```python
from build123d import *
from OCP.BRepFilletAPI import BRepFilletAPI_MakeChamfer

# Parameters (mm, degrees)
BOSS_EXTRUDE1_DEPTH = 16.9
BOSS_EXTRUDE2_DEPTH = 13.5
BOSS_EXTRUDE3_DEPTH = 3.4
BOSS_EXTRUDE4_DEPTH = 13.5
CUT_EXTRUDE1_DEPTH  = 46.31468443
CHAMFER1_SIZE       = 2
CHAMFER1_SIZE2      = 1.154700538
CUT_EXTRUDE2_DEPTH  = 47.441152279
FILLET1_R           = 0.5
SKETCH10_W          = 25
SKETCH10_H          = 28.6
CUT_EXTRUDE3_DEPTH  = 47.441152315


with BuildPart() as part:
    # Sketch1 → Boss-Extrude1 (new body)
    with BuildSketch(Plane.XY):
        Polygon((-20, -13.3), (20, -13.3), (20, 13.3), (-20, 13.3), (-20, 14.3), (21, 14.3), (21, -14.3), (-20, -14.3), align=None)
    extrude(amount=BOSS_EXTRUDE1_DEPTH)

    # Sketch4 → Boss-Extrude2 (add)
    with BuildSketch(Plane(origin=(0, 0, 0), x_dir=(-1, 0, 0), z_dir=(0, 0, -1))):
        with BuildLine():
            Line((-21, 4.825), (-36, 4.825))
            ThreePointArc((-36, 4.825), (-38.610615349, 4.05774722), (-40.390970849, 2))
            Line((-40.390970849, 2), (-30.875, 2))
            Line((-30.875, 2), (-30.875, -2))
            Line((-30.875, -2), (-40.390970849, -2))
            ThreePointArc((-40.390970849, -2), (-38.610615349, -4.05774722), (-36, -4.825))
            Line((-36, -4.825), (-21, -4.825))
            Line((-21, -4.825), (-21, 4.825))
        make_face()
    extrude(amount=-BOSS_EXTRUDE2_DEPTH)

    # Sketch5 → Boss-Extrude3 (add)
    with BuildSketch(Plane.XY.offset(13.5)):
        with BuildLine():
            Line((21, 4.825), (21, -4.825))
            Line((21, -4.825), (36, -4.825))
            ThreePointArc((36, -4.825), (38.610615349, -4.05774722), (40.390970849, -2))
            ThreePointArc((40.390970849, -2), (40.825, 0), (40.390970849, 2))
            ThreePointArc((40.390970849, 2), (38.610615349, 4.05774722), (36, 4.825))
            Line((36, 4.825), (21, 4.825))
        make_face()
    extrude(amount=BOSS_EXTRUDE3_DEPTH)

    # Sketch8 → Boss-Extrude4 (add)
    with BuildSketch(Plane(origin=(0, 0, 0), x_dir=(-1, 0, 0), z_dir=(0, 0, -1))):
        with BuildLine():
            Line((-37.5, 2), (-40.390970849, 2))
            ThreePointArc((-40.390970849, 2), (-40.825, 0), (-40.390970849, -2))
            Line((-40.390970849, -2), (-37.5, -2))
            ThreePointArc((-37.5, -2), (-38.5, 0), (-37.5, 2))
        make_face()
        with BuildLine():
            Line((-34.5, 2), (-30.875, 2))
            Line((-30.875, 2), (-30.875, -2))
            Line((-30.875, -2), (-34.5, -2))
            ThreePointArc((-34.5, -2), (-33.5, 0), (-34.5, 2))
        make_face()
    extrude(amount=-BOSS_EXTRUDE4_DEPTH)

    # Sketch9 → Cut-Extrude1 (cut, through all)
    with BuildSketch(Plane(origin=(0, 0, 13.5), x_dir=(-1, 0, 0), z_dir=(0, 0, -1))):
        with BuildLine():
            Line((-37.5, -2), (-34.5, -2))
            ThreePointArc((-34.5, -2), (-33.5, 0), (-34.5, 2))
            Line((-34.5, 2), (-37.5, 2))
            ThreePointArc((-37.5, 2), (-38.5, 0), (-37.5, -2))
        make_face()
    extrude(amount=-CUT_EXTRUDE1_DEPTH, mode=Mode.SUBTRACT)

    # Chamfer1: one chamfer whose edges measure the first distance from different faces: ONE call of the kernel's chamfer builder (chamfer() names one face for all edges)
    chamfer1_edges_1 = [part.edges().sort_by_distance(p)[0] for p in [
        (36, 2, 0),
    ]]
    chamfer1_side_1 = [part.faces().sort_by_distance(p)[0] for p in [
        (36, 2, 8.45),
    ]]
    chamfer1_edges_2 = [part.edges().sort_by_distance(p)[0] for p in [
        (38.5, 0, 0),
    ]]
    chamfer1_side_2 = [part.faces().sort_by_distance(p)[0] for p in [
        (38.5, 0, 8.45),
    ]]
    chamfer1_edges_3 = [part.edges().sort_by_distance(p)[0] for p in [
        (36, -2, 0),
    ]]
    chamfer1_side_3 = [part.faces().sort_by_distance(p)[0] for p in [
        (36, -2, 8.45),
    ]]
    chamfer1_edges_4 = [part.edges().sort_by_distance(p)[0] for p in [
        (33.5, 0, 0),
    ]]
    chamfer1_side_4 = [part.faces().sort_by_distance(p)[0] for p in [
        (33.5, 0, 8.45),
    ]]
    chamfer1 = BRepFilletAPI_MakeChamfer(part.part.solid().wrapped)
    for e in chamfer1_edges_1:
        chamfer1.Add(CHAMFER1_SIZE, CHAMFER1_SIZE2, e.wrapped, chamfer1_side_1[0].wrapped)  # the first distance lies on this face
    for e in chamfer1_edges_2:
        chamfer1.Add(CHAMFER1_SIZE, CHAMFER1_SIZE2, e.wrapped, chamfer1_side_2[0].wrapped)  # the first distance lies on this face
    for e in chamfer1_edges_3:
        chamfer1.Add(CHAMFER1_SIZE, CHAMFER1_SIZE2, e.wrapped, chamfer1_side_3[0].wrapped)  # the first distance lies on this face
    for e in chamfer1_edges_4:
        chamfer1.Add(CHAMFER1_SIZE, CHAMFER1_SIZE2, e.wrapped, chamfer1_side_4[0].wrapped)  # the first distance lies on this face
    add(Compound.cast(chamfer1.Shape()), mode=Mode.REPLACE)

    # Sketch11 → Cut-Extrude2 (cut, through all)
    with BuildSketch(Plane(origin=(0, 0, 0), x_dir=(-1, 0, 0), z_dir=(0, 0, -1))):
        with BuildLine():
            Line((-34.483424911, 2.05), (-37.516575089, 2.05))
            ThreePointArc((-37.516575089, 2.05), (-38.55, 0), (-37.516575089, -2.05))
            Line((-37.516575089, -2.05), (-34.483424911, -2.05))
            ThreePointArc((-34.483424911, -2.05), (-33.45, 0), (-34.483424911, 2.05))
        make_face()
    extrude(amount=-CUT_EXTRUDE2_DEPTH, mode=Mode.SUBTRACT)

    # Fillet1
    fillet1_edges = [part.edges().sort_by_distance(p)[0] for p in [
        (-20, 14.3, 8.45),
        (21, 14.3, 8.45),
        (21, -14.3, 8.45),
        (-20, -14.3, 8.45),
    ]]
    fillet(fillet1_edges, radius=FILLET1_R)

    # Sketch10 → Cut-Extrude3 (cut, through all)
    with BuildSketch(Plane(origin=(0, 0, 0), x_dir=(-1, 0, 0), z_dir=(0, 0, -1))):
        with Locations((7.5, 0)):
            Rectangle(SKETCH10_W, SKETCH10_H)
    extrude(amount=-CUT_EXTRUDE3_DEPTH, mode=Mode.SUBTRACT)


solid = part.part
```
The listing builds one solid part. Answer for the finished solid, in the listing's coordinates (mm). A direction names the side the tool comes from. Round coordinates to 2 decimals unless told otherwise and drop trailing zeros. Order: outer loops, then holes, each group sorted by start corner. A loop starts at its lowest first (then second) coordinate and runs counter-clockwise, first axis right, second up. Notation, with made-up numbers: (-2.75, -15) - (1.25, -15) arc R9 ccw to (1.25, -2) - close; hole circle Ø4 at (26.5, -25). An arc over 180 degrees is marked (long way). Put each result on its own line as item: value. Start each with the question number.
(1) Find section B-B (z = 8). Give the vertices of the cut face in (x, y) (3 decimals).
(2) Find section C-C (y = 0). Give the vertices of the cut face in (x, z) (3 decimals), plus the area to 3 significant figures.
(3) Straight lines are drawn through the part: probe 1 along Y at (x, z) = (12, 8.75); probe 2 along Y at (x, z) = (35.5, 9.75) (3 decimals); probe 3 along Y at (x, z) = (27.5, 9.75) (3 decimals). For each, find the intervals that lie inside material, in ascending order. Write a range as from..to.
(4) Given P1, Ø4.5, axis at x = 26.5, z = 7.5, coming from the -Y side (3 decimals); P2, Ø2.5, axis at y = 10.5, z = 10, coming from the +X side; P3, Ø0.9, axis at x = 36, z = 9.5, coming from the +Y side (3 decimals), each flat-ended and moving along its own axis, determine where each tip first touches the part or whether it passes through.
(5) Find section D-D (y = 11). Give the vertices of the cut face in (x, z).
(6) For faces 1 (the flat face through (29, 4.825, 8)), 2 (the flat face through (12, -13.3, 8)), 3 (the cylindrical face through (38.55, 0.03, 9.3)), determine the directions among +Z, -Z, +X, -X, +Y, -Y from which every point of the face is accessible in a straight line to the end or side of a thin tool.
(7) Determine the mould class of faces 4 (the flat face through (36.03, 2.61, 0.94)), 5 (the flat face through (13, 13.3, 8)), 6 (the cylindrical face through (40.824, 0.106, 8.332)), 7 (the flat face through (36, 2.05, 9)) for opening direction X: released by +X, released by -X, zero draft, split by the parting line, or undercut.
(8) Find section A-A (x = 9). Give the vertices of the cut face in (y, z).
Reply:
1. outline: (5, -14.3) - (20.5, -14.3) arc R0.5 ccw to (21, -13.8) - (21, -4.825) - (36, -4.825) arc R4.825 ccw to (36, 4.825) - (21, 4.825) - (21, 13.8) arc R0.5 ccw to (20.5, 14.3) - (5, 14.3) - (5, 13.3) - (20, 13.3) - (20, -13.3) - (5, -13.3) - close; hole (34.483, -2.05) - (37.517, -2.05) arc R2.55 ccw to (37.517, 2.05) - (34.483, 2.05) arc R2.55 ccw to start
2. outline: (20, 0) - (32.345, 0) - (33.45, 1.913) - (33.45, 16.9) - (20, 16.9) - close; (38.55, 1.913) - (39.655, 0) - (40.825, 0) - (40.825, 16.9) - (38.55, 16.9) - close
2. area: 264 mm^2
3. probe 1: -14.3..-13.3, 13.3..14.3
3. probe 2: -4.825..-2.05, 2.05..4.825
3. probe 3: -4.825..4.825
4. P1: y = -4.825
4. P2: x = 21
4. P3: y = 4.825
5. outline: (20, 0) - (21, 0) - (21, 16.9) - (20, 16.9) - close
6. face 1: +Z, -Z, +X, +Y
6. face 2: +Z, -Z, -X
6. face 3: +Z, -Z
7. face 4: undercut
7. face 5: zero draft
7. face 6: released by +X
7. face 7: undercut
8. outline: (-14.3, 0) - (-13.3, 0) - (-13.3, 16.9) - (-14.3, 16.9) - close; (13.3, 0) - (14.3, 0) - (14.3, 16.9) - (13.3, 16.9) - close
